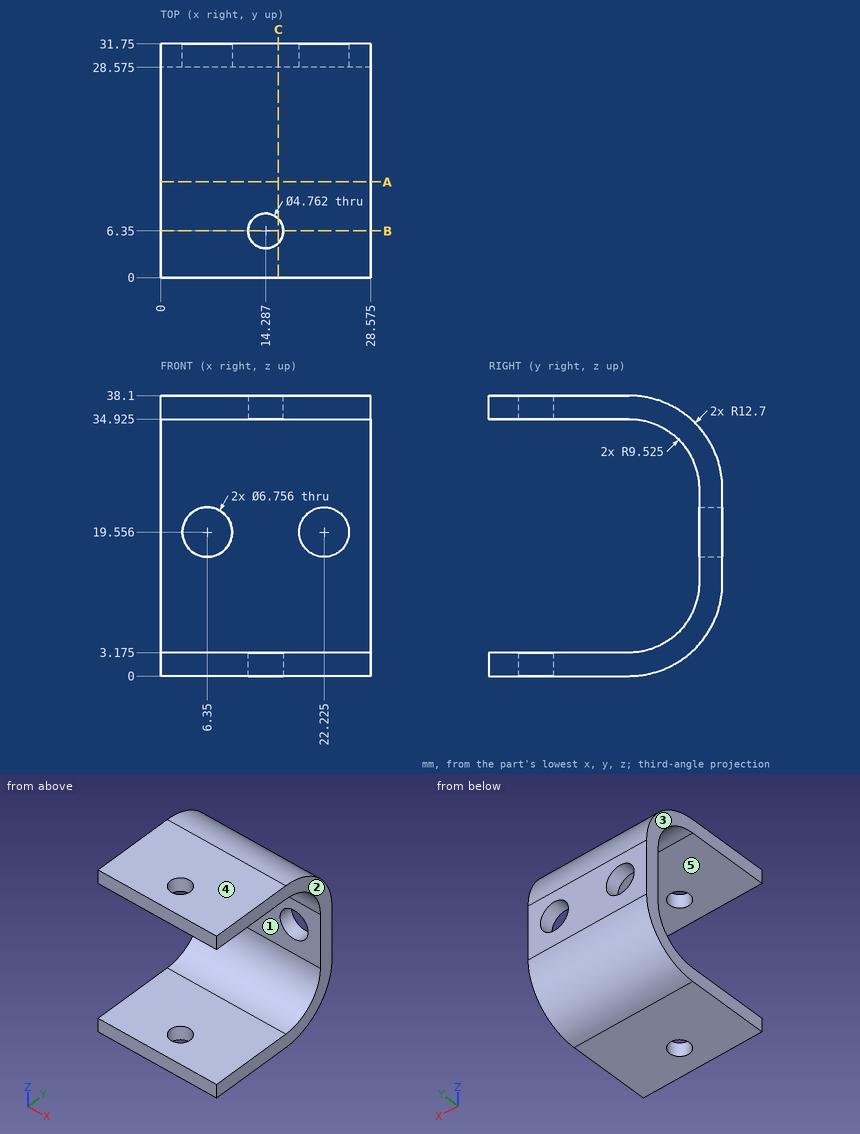
Study the drawing (mm; zero at the part's minimum x, y, z) and answer. A direction names the side the tool comes from. Coordinates: 2 decimals unless noted, no trailing zeros. Write each loop counter-clockwise with the first axis right and the second up, starting at its lowest first coordinate (ties: lowest second). Pieces come first, ordered by that corner, then holes.
Q1. Determine the mould class of the marked faces 3, 4 and 5 for opening direction Z: released by +Z, released by -Z, zero draft, split by the parting line, or undercut.
Q2. A cutting plane is placed at A-A, the plane y = 13. Give the vertices of the cut face in (x, z) (1 decimal).
Q3. Find the intervals of material crossed by line 1 (Z direction, x = 6.5, y = 8.5) (1 decimal); line 2 (X direction, y = 30.5, z = 20.5) (1 decimal); line 3 (Z direction, x = 22.5, y = 24.5), in increasing order.
Q4. Which of the six approach directions +Z, -Z, +X, -X, +Y, -Y give full straight-line access (tool end or side, diameter ignored) to the marked faces 1 and 2?
Q5. A cutting plane is placed at B-B, the plane y = 6.35. Give the vertices of the cut face in (x, z) (1 decimal).
Q6. Each of these flat-tipped pins is pushed along its axis until it touches: pin 1 Ø10 at (x, z) = (15, 22.5) entering from -Y; pin 2 Ø6 at (x, z) = (22.22, 19.56) entering from +Y; pin 3 Ø6 at (x, y) = (14.29, 6.35) entering from +Z; pin 4 Ø4 at (x, z) = (9.5, 16.5) entering from -Y (1 decimal). Where does it stop, or does it pass through?
Q7. A cutting plane is placed at C-C, the plane x = 16. State how many separate pieces and enclosed holes the cut face has, then the cut area to 3 significant figures.
Findings below:
1. face 3: zero draft
1. face 4: released by +Z
1. face 5: undercut
2. outline: (0, 0) - (28.6, 0) - (28.6, 3.2) - (0, 3.2) - close; (0, 34.9) - (28.6, 34.9) - (28.6, 38.1) - (0, 38.1) - close
3. line 1: z = 0 to 3.2, 34.9 to 38.1
3. line 2: x = 0 to 3.1, 9.6 to 19, 25.5 to 28.6
3. line 3: z = 1.23 to 4.89, 33.21 to 36.87
4. face 1: +X, -X, -Y
4. face 2: +Z, -Z, +X, +Y, -Y
5. outline: (0, 0) - (11.9, 0) - (11.9, 3.2) - (0, 3.2) - close; (0, 34.9) - (11.9, 34.9) - (11.9, 38.1) - (0, 38.1) - close; (16.7, 0) - (28.6, 0) - (28.6, 3.2) - (16.7, 3.2) - close; (16.7, 34.9) - (28.6, 34.9) - (28.6, 38.1) - (16.7, 38.1) - close
6. pin 1: stops at y = 28.34
6. pin 2: passes through
6. pin 3: stops at z = 38.1
6. pin 4: stops at y = 28.6
7. separate pieces: 3
7. enclosed holes: 0
7. area: 251 mm2
